from build123d import *

# Parameters (mm, degrees)
BOSS_EXTRU_1_DEPTH      = 1.53
ESQUISSE2_R             = 1.665
ENL_V_MAT_EXTRU_1_DEPTH = 1.53


with BuildPart() as part:
    # Esquisse1 → Boss.-Extru.1 (new body)
    with BuildSketch(Plane.XY):
        with BuildLine():
            Line((0, 7.35), (0, 60.41))
            Line((0, 60.41), (20.31, 60.41))
            Line((20.31, 60.41), (20.31, 7.35))
            Line((20.31, 7.35), (17.0725, 0))
            Line((17.0725, 0), (13.835, 7.35))
            Line((13.835, 7.35), (13.835, 45.25))
            ThreePointArc((13.835, 45.25), (10.155, 48.93), (6.475, 45.25))
            Line((6.475, 45.25), (6.475, 7.35))
            Line((6.475, 7.35), (3.2375, 0))
            Line((3.2375, 0), (0, 7.35))
        make_face()
    extrude(amount=BOSS_EXTRU_1_DEPTH)

    # Esquisse2 → Enlèv. mat.-Extru.1 (cut)
    with BuildSketch(Plane.XY.offset(1.53)):
        with Locations((2.425, 57.885)):
            Circle(ESQUISSE2_R)
        with Locations((17.885, 57.885)):
            Circle(ESQUISSE2_R)
    extrude(amount=-ENL_V_MAT_EXTRU_1_DEPTH, mode=Mode.SUBTRACT)


solid = part.part
Source: CAD feature listing. Evaluate the final solid. Frame: model axes, mm. A direction names the side the tool comes from. Round coordinates to 2 decimals unless told otherwise and drop trailing zeros. Write each loop counter-clockwise with the first axis right and the second up, starting at its lowest first coordinate (ties: lowest second). Pieces come first, ordered by that corner, then holes. Notation, with made-up numbers: (87.25, 6) - (92.25, 6) arc R14 ccw to (92.25, 27) - close; hole circle Ø1 at (-4, -37.75). An arc over 180 degrees is marked (long way). Use CSV: the item, a comma, the result in double quotes. Start each with the question number.
(1) Mould query, pull axis Y, two halves, no side actions, for faces 3 (the face through (5, 4, 1)), 4 (the face through (0, 34, 1)), 5 (the face through (19.423, 57.247, 0.776)), 6 (the face through (3.193, 56.408, 0.776)). Classes: pulls with the +Y half, pulls with the -Y half, needs draft (parallel to the pull), parting line crosses it, or undercut.
(2) Material intervals for probe 1 along X at (y, z) = (8, 0.9) (3 decimals); probe 2 along Y at (x, z) = (2.75, 0.95); probe 3 along Y at (x, z) = (2.25, 0.5), sorted ascending. Write a range as [from, to].
(3) Cut plane C-C, the plane z = 0.25. Give the number of separate pieces and of enclosed holes in the cut face, and give its area (3 significant figures).
(4) First-contact query: pin 1 Ø2 at (x, y) = (2.425, 57.885) entering from -Z. Flat tip, straight axial feed; report the tip coordinate or a pass-through.
(5) Cut plane B-B, the plane x = 18.5. Return loops of the section in (y, z), and give its area (3 significant figures).
(6) Cut plane A-A, the plane y = 15. Return loops of the section in (x, z) (3 decimals), and give its area (3 significant figures).
(7) Cut plane D-D, the plane x = 12. Return loops of the section in (y, z), and give its area (3 significant figures).
(8) Set-up query: faces 1 (the face through (10, 60.41, 1)), 2 (the face through (13.835, 26, 1)). Return all of +Z, -Z, +X, -X, +Y, -Y with unobstructed straight access to the full face (end or side cutting, diameter ignored); none if empty.
Geometry says:
1,face 3,"pulls with the -Y half"
1,face 4,"needs draft"
1,face 5,"undercut"
1,face 6,"undercut"
2,probe 1,"[0, 6.475], [13.835, 20.31]"
2,probe 2,"[1.11, 56.25], [59.52, 60.41]"
2,probe 3,"[2.24, 56.23], [59.54, 60.41]"
3,separate pieces,"1"
3,enclosed holes,"2"
3,area,"808 mm²"
4,pin 1,"through"
5,outline,"(3.24, 0) - (56.34, 0) - (56.34, 1.53) - (3.24, 1.53) - close; (59.43, 0) - (60.41, 0) - (60.41, 1.53) - (59.43, 1.53) - close"
5,area,"82.7 mm²"
6,outline,"(0, 0) - (6.475, 0) - (6.475, 1.53) - (0, 1.53) - close; (13.835, 0) - (20.31, 0) - (20.31, 1.53) - (13.835, 1.53) - close"
6,area,"19.8 mm²"
7,outline,"(48.43, 0) - (60.41, 0) - (60.41, 1.53) - (48.43, 1.53) - close"
7,area,"18.3 mm²"
8,face 1,"+Z, -Z, +X, -X, +Y"
8,face 2,"+Z, -Z, -Y"
